```python
from build123d import *

# Parameters (mm, degrees)
RESSALTO_EXTRUS_O1_DEPTH = 15
ESBO_O3_R                = 2.5
CORTE_EXTRUS_O1_DEPTH    = 15
CHANFRO1_SIZE            = 2
FILETE1_R                = 0.5
CHANFRO5_SIZE            = 2
CHANFRO7_SIZE            = 5
CHANFRO9_SIZE            = 1
CORTE_EXTRUS_O2_DEPTH    = 10
FILETE2_R                = 1


with BuildPart() as part:
    # Esboço1 → Ressalto-extrusão1 (new body)
    with BuildSketch(Plane.XY):
        Polygon((0.299414955, -0.75), (-5.700585045, -0.75), (-5.700585045, -15.95), (14.299414955, -15.95), (14.299414955, -20.95), (-10.700585045, -20.95), (-10.700585045, -0.75), (-110.700585045, -0.75), (-110.700585045, 4.25), (0.299414955, 4.25), align=None)
    extrude(amount=RESSALTO_EXTRUS_O1_DEPTH)

    # Esboço3 → Corte-extrusão1 (cut)
    with BuildSketch(Plane.XZ.offset(20.95)):
        with Locations(Location((6.299414955, 7.5, 0), (0, 0, 270))):
            Circle(ESBO_O3_R)
    extrude(amount=-CORTE_EXTRUS_O1_DEPTH, mode=Mode.SUBTRACT)

    # Chanfro1
    chanfro1_edges = [part.edges().sort_by_distance(p)[0] for p in [
        (6.299414955, -20.95, 10),
    ]]
    chamfer(chanfro1_edges, length=CHANFRO1_SIZE)

    # Filete1
    filete1_edges = [part.edges().sort_by_distance(p)[0] for p in [
        (6.299414955, -15.95, 10),
    ]]
    fillet(filete1_edges, radius=FILETE1_R)

    # Chanfro5
    chanfro5_edges = [part.edges().sort_by_distance(p)[0] for p in [
        (14.299414955, -20.95, 7.5),
        (-10.700585045, -20.95, 7.5),
        (0.299414955, 4.25, 7.5),
    ]]
    chamfer(chanfro5_edges, length=CHANFRO5_SIZE)

    # Chanfro7
    chanfro7_edges = [part.edges().sort_by_distance(p)[0] for p in [
        (-10.700585045, -0.75, 7.5),
    ]]
    chamfer(chanfro7_edges, length=CHANFRO7_SIZE)

    # Chanfro9
    chanfro9_edges = [part.edges().sort_by_distance(p)[0] for p in [
        (13.299414955, -19.95, 0),
        (14.299414955, -17.45, 0),
        (0.299414955, 0.75, 0),
        (-0.700585045, 3.25, 0),
        (-56.200585045, 4.25, 0),
        (-110.700585045, 1.75, 0),
        (-63.200585045, -0.75, 0),
        (-13.200585045, -3.25, 0),
        (-10.700585045, -12.35, 0),
        (-9.700585045, -19.95, 0),
        (1.799414955, -20.95, 0),
        (-110.700585045, 1.75, 15),
        (-56.200585045, 4.25, 15),
        (-0.700585045, 3.25, 15),
        (0.299414955, 0.75, 15),
        (14.299414955, -17.45, 15),
        (13.299414955, -19.95, 15),
        (1.799414955, -20.95, 15),
        (-9.700585045, -19.95, 15),
        (-10.700585045, -12.35, 15),
        (-13.200585045, -3.25, 15),
        (-63.200585045, -0.75, 15),
        (-110.700585045, 4.25, 7.5),
        (-110.700585045, -0.75, 7.5),
    ]]
    chamfer(chanfro9_edges, length=CHANFRO9_SIZE)

    # Esboço4 → Corte-extrusão2 (cut)
    with BuildSketch(Plane.XZ.offset(0.75)):
        with BuildLine():
            Line((-99.700585045, 9.25), (-20.700585045, 9.25))
            ThreePointArc((-20.700585045, 9.25), (-18.950585045, 7.5), (-20.700585045, 5.75))
            Line((-20.700585045, 5.75), (-99.700585045, 5.75))
            ThreePointArc((-99.700585045, 5.75), (-101.450585045, 7.5), (-99.700585045, 9.25))
        make_face()
    extrude(amount=-CORTE_EXTRUS_O2_DEPTH, mode=Mode.SUBTRACT)

    # Filete2
    filete2_edges = [part.edges().sort_by_distance(p)[0] for p in [
        (-101.450585045, 4.25, 7.5),
        (-60.200585045, 4.25, 9.25),
        (-18.950585045, 4.25, 7.5),
        (-60.200585045, 4.25, 5.75),
        (-101.450585045, -0.75, 7.5),
        (-60.200585045, -0.75, 5.75),
        (-18.950585045, -0.75, 7.5),
        (-60.200585045, -0.75, 9.25),
    ]]
    fillet(filete2_edges, radius=FILETE2_R)


solid = part.part
```
The listing builds one solid part. Answer for the finished solid, in the listing's coordinates (mm). A direction names the side the tool comes from. Round coordinates to 2 decimals unless told otherwise and drop trailing zeros. Order: outer loops, then holes, each group sorted by start corner. A loop starts at its lowest first (then second) coordinate and runs counter-clockwise, first axis right, second up. Notation, with made-up numbers: (81.5, -30.75) -> (97.5, -30.75) arc R27 ccw to (97.5, -0.75) -> close; hole circle Ø8 at (86, 20.5). An arc over 180 degrees is marked (long way). Answer as CSV lines item,"result". Start each with the question number.
(1) Find the intervals of material crossed by probe 1 along Z at (x, y) = (-60.5, 1.75); probe 2 along X at (y, z) = (-17.2, 7.5); probe 3 along Y at (x, z) = (-37.5, 11), in increasing order. Write a range as from..to.
(2) The part is cut by section C-C (y = -14.5). Determine the outline of the cut face in (x, z).
(3) A tool of negligible diameter and unlimited length cuts with its end or side. For faces 5 (the face through (12.94, -19.62, 0.51)), 6 (the face through (-10.701, -12, 7)), 7 (the face through (-3, -0.75, 7)), 8 (the face through (0.299, 1, 7)), from which of +Z, -Z, +X, -X, +Y, -Y can it reach the whole face along a straight path? Write none if from no direction.
(4) Flat-ended cylindrical pins translate along their axes: pin 1 Ø7.5 at (y, z) = (-12, 10) entering from +X; pin 2 Ø1.5 at (y, z) = (1, 5.5) entering from +X; pin 3 Ø5 at (x, z) = (-25, 9) entering from -Y. Find the tip coordinate at first contact, or state that the pin passes through.
(5) The part is cut by section B-B (x = -70). Determine the outline of the cut face in (y, z).
(6) The part is cut by section A-A (z = 7.5). Count the separate pieces of the cut face and the enclosed holes in it, then the cut area to 3 significant figures.
(7) For a pull along Z with two mould halves and no side action, classify faces 1 (the face through (-39, 1, 0)), 2 (the face through (-60, 2, 5.75)), 3 (the face through (-18.95, 1.73, 7.54)), 4 (the face through (-5.701, -8, 7)) as +Z half, -Z half, draft (parallel to the pull), parting line (faces both ways), or undercut.
Evaluation:
1,probe 1,"0..5.75, 9.25..15"
1,probe 2,"-10.7..3.8, 8.8..14.3"
1,probe 3,"-0.75..4.25"
2,outline,"(-10.7, 1) -> (-9.7, 0) -> (-5.7, 0) -> (-5.7, 15) -> (-9.7, 15) -> (-10.7, 14) -> close"
3,face 5,"-Z, +X, -Y"
3,face 6,"+Z, -Z, -X, -Y"
3,face 7,"+Z, -Z, +X"
3,face 8,"+Z, -Z, +X, +Y"
4,pin 1,"x = -5.7"
4,pin 2,"x = 0.3"
4,pin 3,"y = -0.75"
5,outline,"(-0.75, 1) -> (0.25, 0) -> (3.25, 0) -> (4.25, 1) -> (4.25, 4.75) arc R1 ccw to (3.25, 5.75) -> (0.25, 5.75) arc R1 ccw to (-0.75, 4.75) -> close; (-0.75, 10.25) arc R1 ccw to (0.25, 9.25) -> (3.25, 9.25) arc R1 ccw to (4.25, 10.25) -> (4.25, 14) -> (3.25, 15) -> (0.25, 15) -> (-0.75, 14) -> close"
6,separate pieces,"3"
6,enclosed holes,"0"
6,area,"319 mm²"
7,face 1,"-Z half"
7,face 2,"undercut"
7,face 3,"undercut"
7,face 4,"draft"
